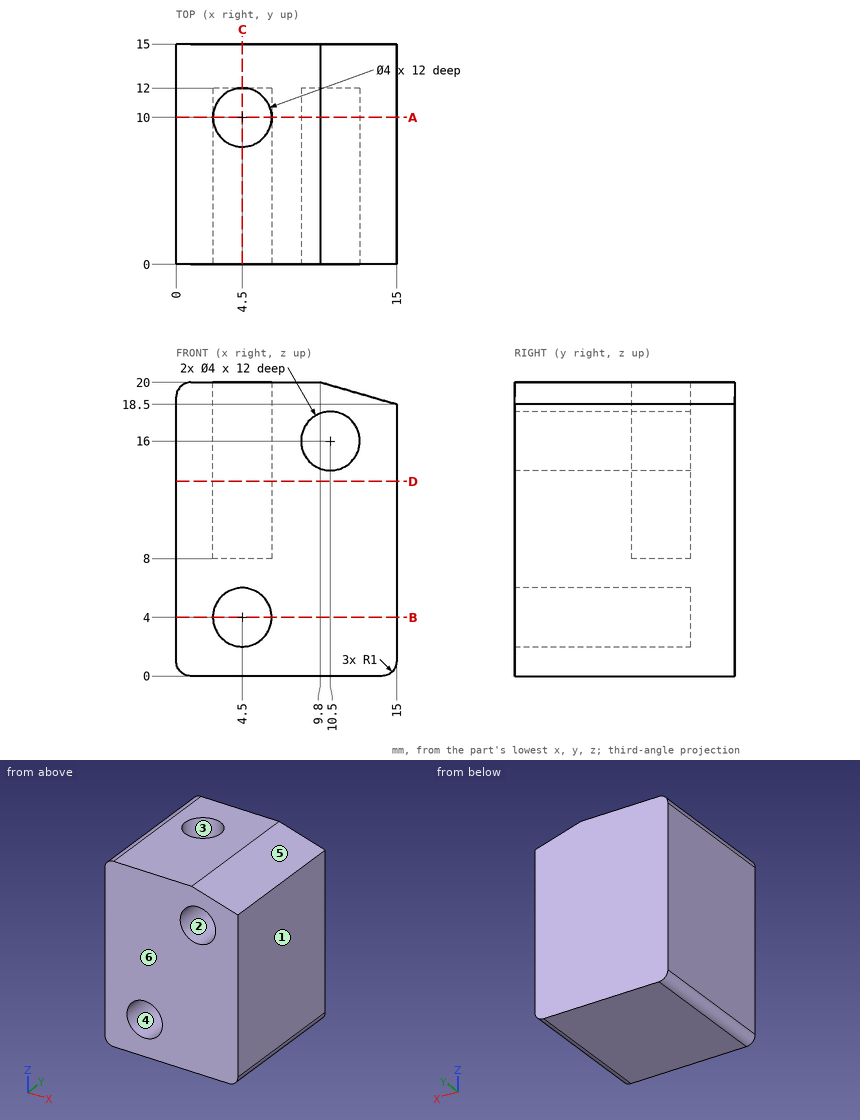
The figure shows three views and two pictorial views of one solid part (mm, origin at its lowest corner). Answer the questions. A direction names the side the tool comes from. Coordinates: 2 decimals unless noted, no trailing zeros. Loops run counter-clockwise (first coordinate to the right, second up) from the corner with the lowest first, then second, coordinate; pieces in that order, holes last. Notation, with made-up numbers: (-14, 46.5) - (-1, 46.5) arc R22 cw to (-1, 78.5) - close; hole circle Ø5 at (88.25, 80.25). An arc over 180 degrees is marked (long way). Answer in a Markdown table with one row per item.
Q1. Straight lines are drawn through the part: line 1 along X through (y, z) = (8.25, 16); line 2 along X through (y, z) = (6.5, 4); line 3 along Z through (x, y) = (3.5, 2). For each, find the intervals that lie inside material, in ascending order. Write a range as [from, to].
Here are the results:
| item | result |
|---|---|
| line 1 | x = [0, 3.53], [5.47, 8.5], [12.5, 15] |
| line 2 | x = [0, 2.5], [6.5, 15] |
| line 3 | z = [0, 2.27], [5.73, 20] |
Q2. Find section C-C on x = 4.5. Write down the section's boundary in (y, z), plus the area to 3 significant figures.
Here are the results:
| item | result |
|---|---|
| outline | (0, 0) - (15, 0) - (15, 20) - (12, 20) - (12, 8) - (8, 8) - (8, 20) - (0, 20) - (0, 6) - (12, 6) - (12, 2) - (0, 2) - close |
| area | 204 mm^2 |
Q3. Given P1, Ø1.2, axis at x = 4, y = 9.5, coming from the +Z side; P2, Ø5, axis at x = 10.5, z = 16, coming from the -Y side; P3, Ø3.5, axis at x = 4.5, z = 4, coming from the -Y side, each flat-ended and moving along its own axis, determine where each tip first touches the part or whether it passes through.
Here are the results:
| item | result |
|---|---|
| P1 | stops at z = 8 |
| P2 | stops at y = 0 |
| P3 | stops at y = 12 |
Q4. Find section B-B on z = 4. Write down the section's boundary in (x, y).
Here are the results:
| item | result |
|---|---|
| outline | (0, 0) - (2.5, 0) - (2.5, 12) - (6.5, 12) - (6.5, 0) - (15, 0) - (15, 15) - (0, 15) - close |
Q5. Find section A-A on y = 10. Write down the section's boundary in (x, z).
Here are the results:
| item | result |
|---|---|
| outline | (0, 1) arc R1 ccw to (1, 0) - (14, 0) arc R1 ccw to (15, 1) - (15, 18.5) - (9.8, 20) - (6.5, 20) - (6.5, 8) - (2.5, 8) - (2.5, 20) - (1, 20) arc R1 ccw to (0, 19) - close; hole circle Ø4 at (4.5, 4); hole circle Ø4 at (10.5, 16) |
Q6. Find section D-D on z = 13.25. Write down the section's boundary in (x, y).
Here are the results:
| item | result |
|---|---|
| outline | (0, 0) - (15, 0) - (15, 15) - (0, 15) - close; hole circle Ø4 at (4.5, 10) |
Q7. For the marked faces 1, 2 and 3, determine the directions among +Z, -Z, +X, -X, +Y, -Y from which every point of the face is accessible in a straight line to the end or side of a thin tool.
Here are the results:
| item | result |
|---|---|
| face 1 | +Z, -Z, +X, +Y, -Y |
| face 2 | -Y |
| face 3 | +Z |
Q8. The mould has two halves that part along X. Classify the marked faces 4, 5 and 6: pulls with the +X half, pulls with the -X half, needs draft (parallel to the pull), parting line crosses it, or undercut.
Here are the results:
| item | result |
|---|---|
| face 4 | undercut |
| face 5 | pulls with the +X half |
| face 6 | needs draft |
